Can you work these out from the model? Positions are in its coordinate system, mm. A direction names the side the tool comes from. Round coordinates to 2 decimals unless told otherwise and drop trailing zeros. Write each loop counter-clockwise with the first axis right and the second up, starting at its lowest first coordinate (ties: lowest second). Pieces come first, ordered by that corner, then holes. Notation, with made-up numbers: (78.25, 64.25) - (103.25, 64.25) arc R27 cw to (103.25, 81.25) - close; hole circle Ø6 at (3, 73.25). An arc over 180 degrees is marked (long way). One line per item, written item: value. Start each with the question number.
(1) If I drill on L1, parallel to X at y = 25, z = 3.5; L2, parallel to X at y = -31.5, z = 9.5; L3, parallel to Y at x = 49, z = 8.5, over which ranges is the centre line in solid material (lowest first)? Write a range as from..to.
(2) I'm going to push flat-ended pins straight in: pin 1 Ø8 at (x, y) = (8.5, -8.87) entering from -Z; pin 2 Ø3 at (y, z) = (21.5, 7.5) entering from +X. Where does each tip first touch, or does it pass through?
(3) I want a section at B-B on x = 61. List the corners of the cut face in (y, z) for me, plus the area to 3 significant figures.
(4) On a 3-axis mill with a long thin cutter (end or side, diameter ignored), from which of +Z, -Z, +X, -X, +Y, -Y can I reach the whole of each face in a straight line? I mean faces 1 (the face through (54.474, 8.034, 4.93)), 2 (the face through (-17.86, 28.63, 7.05)). Say none if no direction works.
(5) I want a section at A-A on z = 8.25. List the corners of the cut face in (x, y) for me, plus the area to 3 significant figures.
(6) I want a section at C-C on y = -14. List the corners of the cut face in (x, z) for me.
(7) Thinking about a two-plate mould opening in Z: for faces 3 (the face through (20, -12, 0)), 4 (the face through (45.085, -30.615, 4.93)), 5 (the face through (29.35, 28.63, 6.28)), which applies, +Z half, -Z half, draft (parallel to the pull), parting line (faces both ways), or undercut?
from build123d import *

# Parameters (mm, degrees)
BOSS_EXTRUDE1_DEPTH   = 10
M6_TAPPED_HOLE1_D     = 5
M6_TAPPED_HOLE1_DEPTH = 15
M6_TAPPED_HOLE1_TIP   = 1.502151548
M5_TAPPED_HOLE1_D     = 4.2
M5_TAPPED_HOLE1_DEPTH = 8
M5_TAPPED_HOLE1_TIP   = 1.2618073


with BuildPart() as part:
    # Sketch2 → Boss-Extrude1 (new body)
    with BuildSketch(Plane.XY):
        Polygon((39.684210526, 32.684210526), (69.684210526, -17.315789474), (69.684210526, -57.315789474), (-30.315789474, -57.315789474), (-30.315789474, 32.684210526), align=None)
    extrude(amount=BOSS_EXTRUDE1_DEPTH)

    # M6 Tapped Hole1
    with Locations(Plane.XY.offset(10)):
        with Locations((8.498638941, -8.865789474), (47.469782111, -31.365789474), (27.984210526, -20.115789474)):
            Hole(M6_TAPPED_HOLE1_D / 2, depth=M6_TAPPED_HOLE1_DEPTH)
            with Locations((0, 0, -(M6_TAPPED_HOLE1_DEPTH + M6_TAPPED_HOLE1_TIP / 2))):  # 118° drill point
                Cone(0, M6_TAPPED_HOLE1_D / 2, M6_TAPPED_HOLE1_TIP, mode=Mode.SUBTRACT)

    # M5 Tapped Hole1
    with Locations(Plane(origin=(0, 32.684210526, 0), x_dir=(1, 0, 0), z_dir=(0, 1, 0))):
        with Locations((-18.315789474, -5), (27.684210526, -5)):
            Hole(M5_TAPPED_HOLE1_D / 2, depth=M5_TAPPED_HOLE1_DEPTH)
            with Locations((0, 0, -(M5_TAPPED_HOLE1_DEPTH + M5_TAPPED_HOLE1_TIP / 2))):  # 118° drill point
                Cone(0, M5_TAPPED_HOLE1_D / 2, M5_TAPPED_HOLE1_TIP, mode=Mode.SUBTRACT)


solid = part.part
Established:
1. L1: -30.32..-19.79, -16.85..26.21, 29.15..44.29
1. L2: -30.32..44.97, 49.97..69.68
1. L3: -57.32..-33.34, -29.39..17.16
2. pin 1: z = 0
2. pin 2: x = 47.29
3. outline: (-57.32, 0) - (-2.84, 0) - (-2.84, 10) - (-57.32, 10) - close
3. area: 545 mm2
4. face 1: +Z, -Z, +X, +Y
4. face 2: +Y
5. outline: (-30.32, -57.32) - (69.68, -57.32) - (69.68, -17.32) - (39.68, 32.68) - (-30.32, 32.68) - close; hole circle Ø5 at (8.5, -8.87); hole circle Ø5 at (27.98, -20.12); hole circle Ø5 at (47.47, -31.37)
5. area: 8,190 mm2
6. outline: (-30.32, 0) - (67.69, 0) - (67.69, 10) - (-30.32, 10) - close
7. face 3: -Z half
7. face 4: draft
7. face 5: undercut
